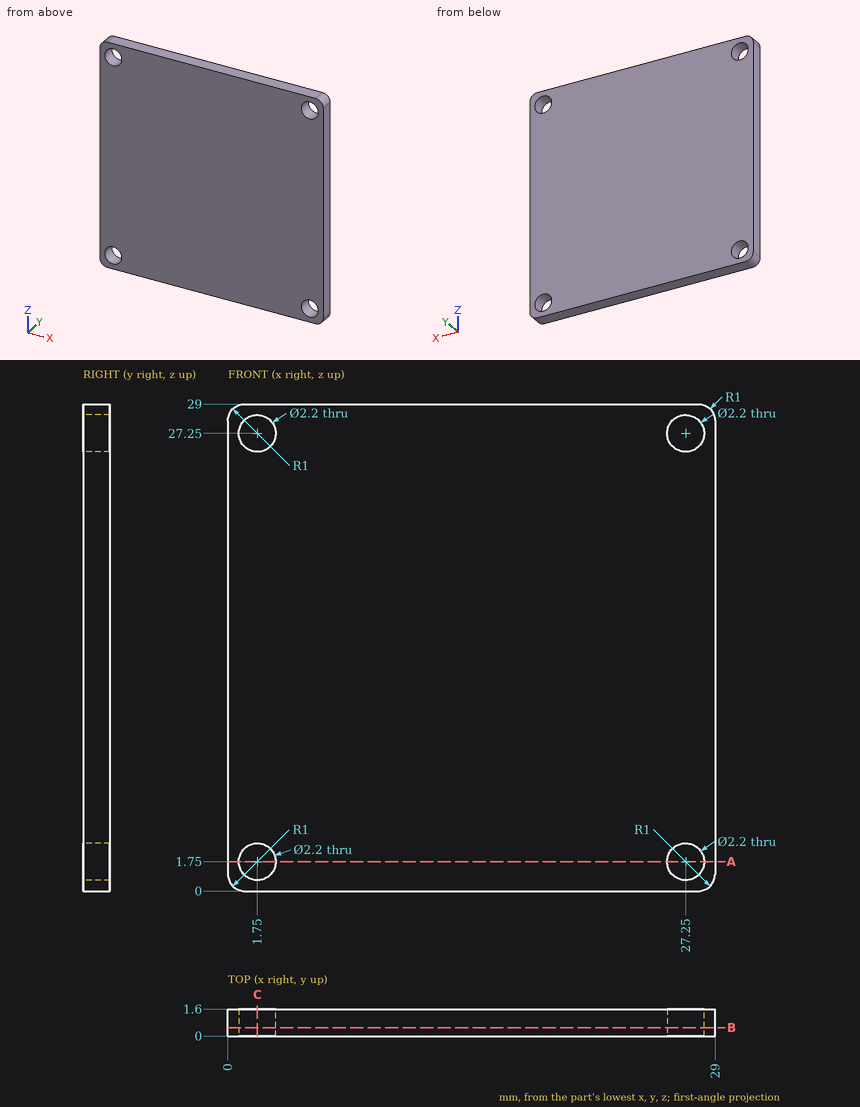
Can you work these out from the drawing? Everything is in mm from the part's minimum corner. Round coordinates to 2 decimals unless told otherwise and drop trailing zeros. Order: outer loops, then holes, each group sorted by start corner. A loop starts at its lowest first (then second) coordinate and runs counter-clockwise, first axis right, second up. Notation, with made-up numbers: (-36, 47) -> (7, 47) arc R18 ccw to (7, 73) -> close; hole circle Ø1 at (-12.75, -0.5). An arc over 180 degrees is marked (long way). Return JSON: item names as keys, results as strings. Group by question number.
1. Will this pin go through, and if not, where does the flat tip stop? pin 1 (2 mm diameter, centred on x = 1.75, z = 27.25, fed in from -Y).
2. If we section it at B-B, the plane y = 0.5: Write out the boundary of the cut face in (x, z), then the cut area to 3 significant figures.
3. I need wall thicknesses on line 1 (X direction, y = 0.55, z = 1.75). Which ranges of the line are inside material? Lowest first, please. Write a range as [from, to].
4. If we section it at A-A, the plane z = 1.75: Write out the boundary of the cut face in (x, y).
5. If we section it at C-C, the plane x = 1.75: Write out the boundary of the cut face in (y, z).
Output values:
{
 "1": {"pin 1": "through"},
 "2": {"outline": "(0, 1) arc R1 ccw to (1, 0) -> (28, 0) arc R1 ccw to (29, 1) -> (29, 28) arc R1 ccw to (28, 29) -> (1, 29) arc R1 ccw to (0, 28) -> close; hole circle Ø2.2 at (1.75, 1.75); hole circle Ø2.2 at (1.75, 27.25); hole circle Ø2.2 at (27.25, 1.75); hole circle Ø2.2 at (27.25, 27.25)", "area": "825 mm²"},
 "3": {"line 1": "[0, 0.65], [2.85, 26.15], [28.35, 29]"},
 "4": {"outline": "(0, 0) -> (0.65, 0) -> (0.65, 1.6) -> (0, 1.6) -> close; (2.85, 0) -> (26.15, 0) -> (26.15, 1.6) -> (2.85, 1.6) -> close; (28.35, 0) -> (29, 0) -> (29, 1.6) -> (28.35, 1.6) -> close"},
 "5": {"outline": "(0, 0) -> (1.6, 0) -> (1.6, 0.65) -> (0, 0.65) -> close; (0, 2.85) -> (1.6, 2.85) -> (1.6, 26.15) -> (0, 26.15) -> close; (0, 28.35) -> (1.6, 28.35) -> (1.6, 29) -> (0, 29) -> close"}
}
